from build123d import *

# Parameters (mm, degrees)
SKETCH1_R      = 10
EXTRUDE1_DEPTH = 10
SKETCH2_R      = 3.9
EXTRUDE2_DEPTH = 10.2
EXTRUDE3_REACH = 26.658
SKETCH3_R      = 2.6


with BuildPart() as part:
    # Sketch1 → Extrude1 (new body)
    with BuildSketch(Plane.XY):
        Circle(SKETCH1_R)
    extrude(amount=EXTRUDE1_DEPTH)

    # Sketch2 → Extrude2 (add)
    with BuildSketch(Plane.XY.offset(10)):
        Circle(SKETCH2_R)
    extrude(amount=EXTRUDE2_DEPTH)

    # Sketch3 → Extrude3 (cut, up to next)
    with BuildSketch(Plane.XY.offset(20.2), mode=Mode.PRIVATE) as extrude3_sk1:
        Circle(SKETCH3_R)
    extrude3_tool1 = extrude(extrude3_sk1.sketch, amount=-EXTRUDE3_REACH, mode=Mode.PRIVATE) & part.part
    add(extrude3_tool1.solids().sort_by_distance((0, 0, 20.2))[0], mode=Mode.SUBTRACT)


solid = part.part
Verification items for the finished model (mm, model axes). A direction names the side the tool comes from. Coordinates: 2 decimals unless noted, no trailing zeros. Order: outer loops, then holes, each group sorted by start corner. A loop starts at its lowest first (then second) coordinate and runs counter-clockwise, first axis right, second up. Notation, with made-up numbers: M 30.5,80 L 63.5,80 A21 ccw 63.5,102 Z; hole C -20.5,15.5 d3. An arc over 180 degrees is marked long. Write each question's results on one line, items separated by ' | '.
1) Gauge pin test, flat ends, axial feed: pin 1 Ø2 at (x, y) = (-7.5, 1.5) entering from -Z; pin 2 Ø6 at (x, z) = (2.5, 12.5) entering from -Y; pin 3 Ø10 at (x, y) = (8, 8) entering from +Z; pin 4 Ø1.5 at (y, z) = (5.5, 10) entering from +X. Record the tip position at first contact, or that the pin passes through.
Solved:
pin 1: stops at z = 0 | pin 2: stops at y = -9.96 | pin 3: stops at z = 10 | pin 4: stops at x = 8.8
2) Section check A-A on x = 0. Record the cut outline in (y, z), plus the area to 3 significant figures.
Solved:
outline: M -10,0 L -2.6,0 L -2.6,20.2 L -3.9,20.2 L -3.9,10 L -10,10 Z; M 2.6,0 L 10,0 L 10,10 L 3.9,10 L 3.9,20.2 L 2.6,20.2 Z | area: 175 mm²
3) Section check D-D on y = 3.5. Record the cut outline in (x, z).
Solved:
outline: M -9.37,0 L 9.37,0 L 9.37,10 L 1.72,10 L 1.72,20.2 L -1.72,20.2 L -1.72,10 L -9.37,10 Z
4) Section check C-C on z = 13.75. Record the cut outline in (x, y), plus the area to 3 significant figures.
Solved:
outline: C 0,0 d7.8; hole C 0,0 d5.2 | area: 26.5 mm²
5) Scan lines: line 1 along Y through (x, z) = (0, 9.25); line 2 along Y through (x, z) = (0, 14.5); line 3 along Z through (x, y) = (-4.75, 7.25). Record each from-to range of solid material in increasing order. Write a range as [from, to].
Solved:
line 1: y = [-10, -2.6], [2.6, 10] | line 2: y = [-3.9, -2.6], [2.6, 3.9] | line 3: z = [0, 10]
6) Access from +Z, -Z, +X, -X, +Y, -Y to the whole of each face (thin tool, end or side, straight path). Record for faces 4 (the face through (2, -2, 0)), 5 (the face through (-2.87, 2.64, 15.03)).
Solved:
face 4: -Z, +X, -X, +Y, -Y | face 5: +Z
7) Release check for a two-part mould opening along X. For faces 1 (the face through (-0.338, 2.578, 10.241)), 2 (the face through (-2.17, -9.76, 4.93)), 3 (the face through (3, -1, 20.2)) record: pulls with the +X half, pulls with the -X half, needs draft (parallel to the pull), parting line crosses it, or undercut.
Solved:
face 1: undercut | face 2: parting line crosses it | face 3: needs draft
